The model under review builds one solid part; all positions refer to its coordinate system, in mm. A direction names the side the tool comes from. Round coordinates to 2 decimals unless told otherwise and drop trailing zeros. Order: outer loops, then holes, each group sorted by start corner. A loop starts at its lowest first (then second) coordinate and runs counter-clockwise, first axis right, second up.
```python
from build123d import *

# Parameters (mm, degrees)
SKETCH1_W           = 107
SKETCH1_H           = 87.7
BOSS_EXTRUDE1_DEPTH = 13.85
SKETCH2_W           = 102.38
SKETCH2_H           = 83.08
CUT_EXTRUDE1_DEPTH  = 7.9
CUT_EXTRUDE2_DEPTH  = 4
SKETCH4_R           = 2.5
SKETCH4_R_2         = 1.2
BOSS_EXTRUDE2_DEPTH = 6.2
SKETCH5_W           = 28
SKETCH5_H           = 2.7
CUT_EXTRUDE3_DEPTH  = 3.5
CHAMFER1_SIZE       = 2
SKETCH6_W           = 8
SKETCH6_H           = 9.85
CUT_EXTRUDE4_DEPTH  = 2.31
SKETCH7_W           = 11.25
SKETCH7_H           = 4.8
BOSS_EXTRUDE3_DEPTH = 1.7
BOSS_EXTRUDE4_DEPTH = 3.15


with BuildPart() as part:
    # Sketch1 → Boss-Extrude1 (new body)
    with BuildSketch(Plane(origin=(0, 0, 0), x_dir=(1, 0, 0), z_dir=(0, 1, 0))):
        Rectangle(SKETCH1_W, SKETCH1_H)
    extrude(amount=BOSS_EXTRUDE1_DEPTH)

    # Sketch2 → Cut-Extrude1 (cut)
    with BuildSketch(Plane(origin=(0, 13.85, 0), x_dir=(1, 0, 0), z_dir=(0, 1, 0))):
        Rectangle(SKETCH2_W, SKETCH2_H)
    extrude(amount=-CUT_EXTRUDE1_DEPTH, mode=Mode.SUBTRACT)

    # Sketch3 → Cut-Extrude2 (cut)
    with BuildSketch(Plane.XZ):
        Polygon((-51.19, 41.54), (51.19, 41.54), (51.19, 19.24), (23.5, 19.24), (23.5, 14.74), (49.4, 14.74), (49.4, 17.44), (53.5, 17.44), (53.5, -20.56), (51.19, -20.56), (51.19, -41.54), (10.19, -41.54), (10.19, -22.86), (40.69, -22.86), (42.704360061, -23.54), (43.44, -21.360818071), (41.067741267, -20.56), (6.19, -20.56), (6.19, -43.85), (-6.19, -43.85), (-6.19, -20.56), (-41.067741267, -20.56), (-43.44, -21.360818071), (-42.704360061, -23.54), (-40.69, -22.86), (-10.19, -22.86), (-10.19, -41.54), (-51.19, -41.54), (-51.19, -20.56), (-53.5, -20.56), (-53.5, 17.44), (-49.4, 17.44), (-49.4, 14.74), (-23.5, 14.74), (-23.5, 19.24), (-51.19, 19.24), align=None)
    extrude(amount=-CUT_EXTRUDE2_DEPTH, mode=Mode.SUBTRACT)

    # Sketch4 → Boss-Extrude2 (add)
    with BuildSketch(Plane(origin=(0, 5.95, 0), x_dir=(1, 0, 0), z_dir=(0, 1, 0))):
        with Locations((-42.5, -25)):
            Circle(SKETCH4_R)
        with Locations((-42.5, -25)):
            Circle(SKETCH4_R_2, mode=Mode.SUBTRACT)
        with Locations((42.5, 25)):
            Circle(SKETCH4_R)
        with Locations((42.5, 25)):
            Circle(SKETCH4_R_2, mode=Mode.SUBTRACT)
    extrude(amount=BOSS_EXTRUDE2_DEPTH)

    # Sketch5 → Cut-Extrude3 (cut)
    with BuildSketch(Plane(origin=(0, 5.95, 0), x_dir=(1, 0, 0), z_dir=(0, 1, 0))):
        with Locations((-36.36, -16.09)):
            Rectangle(SKETCH5_W, SKETCH5_H)
        with Locations((36.36, -16.09)):
            Rectangle(SKETCH5_W, SKETCH5_H)
    extrude(amount=-CUT_EXTRUDE3_DEPTH, mode=Mode.SUBTRACT)

    # Chamfer1
    chamfer1_edges = [part.edges().sort_by_distance(p)[0] for p in [
        (-36.45, 2.45, 14.74),
        (36.45, 2.45, 14.74),
    ]]
    chamfer(chamfer1_edges, length=CHAMFER1_SIZE)

    # Sketch6 → Cut-Extrude4 (cut)
    with BuildSketch(Plane.ZY.offset(53.5)):
        with Locations((0, 8.925)):
            Rectangle(SKETCH6_W, SKETCH6_H)
    cut_extrude4 = extrude(amount=-CUT_EXTRUDE4_DEPTH, mode=Mode.SUBTRACT)

    # Sketch7 → Boss-Extrude3 (add)
    with BuildSketch(Plane(origin=(-51.19, 0, 0), x_dir=(0, 0, -1), z_dir=(1, 0, 0))):
        with Locations((0, 8.35)):
            Rectangle(SKETCH7_W, SKETCH7_H)
    boss_extrude3 = extrude(amount=BOSS_EXTRUDE3_DEPTH)

    # Sketch8 → Boss-Extrude4 (add, symmetric)
    with BuildSketch(Plane.XY):
        Polygon((-49.49, 10.75), (-49.49, 18.75), (-50.99, 18.75), (-51.99, 16.75), (-51.19, 16.75), (-51.19, 10.75), align=None)
    boss_extrude4 = extrude(amount=BOSS_EXTRUDE4_DEPTH, both=True)

    # Mirror1: Cut-Extrude4, Boss-Extrude3, Boss-Extrude4 across plane
    add(cut_extrude4.mirror(Plane(origin=(0, 0, 0), x_dir=(0, 0, 1), z_dir=(1, 0, 0))), mode=Mode.SUBTRACT)
    add(boss_extrude3.mirror(Plane(origin=(0, 0, 0), x_dir=(0, 0, 1), z_dir=(1, 0, 0))))
    add(boss_extrude4.mirror(Plane(origin=(0, 0, 0), x_dir=(0, 0, 1), z_dir=(1, 0, 0))))


solid = part.part
```
(1) Consider section B-B (z = -25). Write out the cut boundary in (x, y), and give its area (3 significant figures).
Data:
outline: (-53.5, 0) - (-51.19, 0) - (-51.19, 4) - (-10.19, 4) - (-10.19, 0) - (-6.19, 0) - (-6.19, 4) - (6.19, 4) - (6.19, 0) - (10.19, 0) - (10.19, 4) - (51.19, 4) - (51.19, 0) - (53.5, 0) - (53.5, 13.85) - (51.19, 13.85) - (51.19, 5.95) - (45, 5.95) - (45, 12.15) - (43.7, 12.15) - (43.7, 5.95) - (41.3, 5.95) - (41.3, 12.15) - (40, 12.15) - (40, 5.95) - (-51.19, 5.95) - (-51.19, 13.85) - (-53.5, 13.85) - close
area: 312 mm2
(2) For faces 1 (the flat face through (-52, 9, 4)), 2 (the flat face through (-1, 10, -41.54)), 3 (the flat face through (-51.19, 2, -31)), 4 (the flat face through (-50, 15, -3.15)), list the 3-axis set-ups (+Z, -Z, +X, -X, +Y, -Y) from which the entire face can be reached by the end or side of a thin tool; tool diameter is ignored.
Data:
face 1: -X, +Y, -Y
face 2: +Y
face 3: -Y
face 4: +X, -X, +Y
(3) Consider section C-C (x = 0). Write out the cut boundary in (y, z).
Data:
outline: (0, 41.54) - (4, 41.54) - (4, -43.85) - (13.85, -43.85) - (13.85, -41.54) - (5.95, -41.54) - (5.95, 41.54) - (13.85, 41.54) - (13.85, 43.85) - (0, 43.85) - close
(4) Consider section A-A (x = 29). Write out the cut boundary in (y, z).
Data:
outline: (0, -43.85) - (13.85, -43.85) - (13.85, -41.54) - (5.95, -41.54) - (5.95, 14.74) - (4, 14.74) - (4, -20.56) - (0, -20.56) - (0, -22.86) - (4, -22.86) - (4, -41.54) - (0, -41.54) - close; (0, 14.74) - (0.45, 14.74) - (2.45, 16.74) - (2.45, 17.44) - (5.95, 17.44) - (5.95, 41.54) - (13.85, 41.54) - (13.85, 43.85) - (0, 43.85) - (0, 41.54) - (4, 41.54) - (4, 19.24) - (0, 19.24) - close
(5) Draft analysis for pull direction Z (two halves, no side actions). For faces 5 (the flat face through (-1, 7, 43.85)), 6 (the flat face through (51.19, 2, -31)), 7 (the flat face through (0, 13.85, 42)), state which applies: pulls with the +Z half, pulls with the -Z half, needs draft (parallel to the pull), parting line crosses it, or undercut.
Data:
face 5: pulls with the +Z half
face 6: undercut
face 7: needs draft
(6) Consider section D-D (z = -10.5). Write out the cut boundary in (x, y), and give its area (3 significant figures).
Data:
outline: (-53.5, 4) - (53.5, 4) - (53.5, 13.85) - (51.19, 13.85) - (51.19, 5.95) - (-51.19, 5.95) - (-51.19, 13.85) - (-53.5, 13.85) - close
area: 245 mm2
(7) To check wall thickness, follow probe 1 along Z at (x, y) = (42.5, 8); probe 2 along Z at (x, y) = (-42.5, 9.5); probe 3 along X at (y, z) = (8.5, 25). State the ranges of each line that lie inside material, in increasing order.
Data:
probe 1: z = -43.85 to -41.54, -27.5 to -26.2, -23.8 to -22.5, 41.54 to 43.85
probe 2: z = -43.85 to -41.54, 22.5 to 23.8, 26.2 to 27.5, 41.54 to 43.85
probe 3: x = -53.5 to -51.19, -45 to -43.7, -41.3 to -40, 51.19 to 53.5
(8) Insertion check: pin 1 (6 mm diameter, centred on x = -26.5, z = 5.5, fed in from +Y); pin 2 (3 mm diameter, centred on x = 42.5, z = -25, fed in from +Y). Each pin has a flat end and moves straight along its axis. Give the tip position at first contact, or say it passes through.
Data:
pin 1: stops at y = 5.95
pin 2: stops at y = 12.15
